Source: three-view drawing plus pictorial views. Frame: mm from the lowest corner of the part. Give positions to 0.01 mm unless a question says otherwise; leave off trailing zeros. Loops run counter-clockwise (first coordinate to the right, second up) from the corner with the lowest first, then second, coordinate; pieces in that order, holes last.
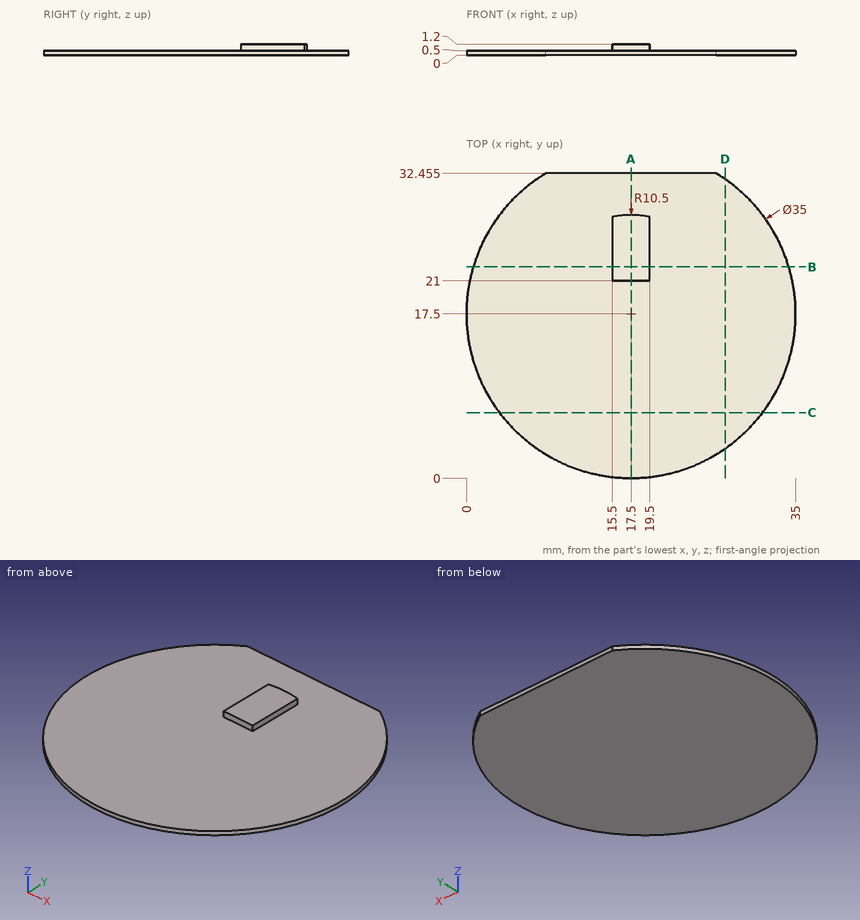
1) Contact query for flat-ended pins moving along their axis: P1, Ø12, axis at x = 25.5, y = 18, coming from the -Z side; P2, Ø0.6, axis at y = 23.5, z = 1, coming from the +X side; P3, Ø8, axis at x = 27, y = 25, coming from the +Z side. Output: stop coordinate, or through.
Checks:
P1: stops at z = 0
P2: stops at x = 19.5
P3: stops at z = 0.5
2) Ray query, probe 1 along Z at (x, y) = (14, 30); probe 2 along Y at (x, z) = (18, 0.4) (1 decimal); probe 3 along X at (y, z) = (27, 1.1). Return the intervals inside material, ascending.
Checks:
probe 1: z = 0 to 0.5
probe 2: y = 0 to 32.5
probe 3: x = 15.5 to 19.5
3) Cut plane A-A (x = 17.5). Return loops of the section in (y, z) (1 decimal).
Checks:
outline: (0, 0) - (32.5, 0) - (32.5, 0.5) - (28, 0.5) - (28, 1.2) - (21, 1.2) - (21, 0.5) - (0, 0.5) - close
4) Cut plane C-C (y = 7). Return loops of the section in (x, z).
Checks:
outline: (3.5, 0) - (31.5, 0) - (31.5, 0.5) - (3.5, 0.5) - close
5) Cut plane B-B (y = 22.5). Return loops of the section in (x, z).
Checks:
outline: (0.73, 0) - (34.27, 0) - (34.27, 0.5) - (19.5, 0.5) - (19.5, 1.2) - (15.5, 1.2) - (15.5, 0.5) - (0.73, 0.5) - close
6) Cut plane D-D (x = 27.5). Return loops of the section in (y, z).
Checks:
outline: (3.14, 0) - (31.86, 0) - (31.86, 0.5) - (3.14, 0.5) - close
